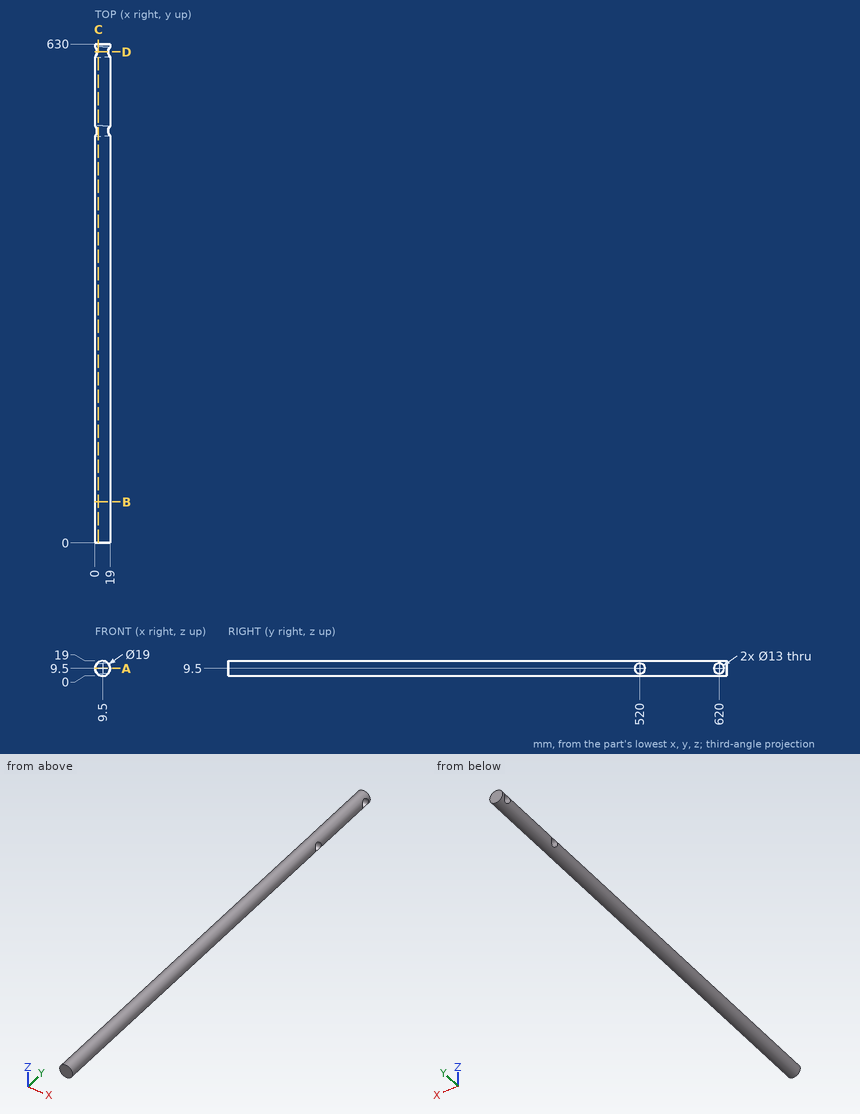
Geometry check sheet. Reference: drawing and pictorial views, mm from the part's lowest x, y, z. Round coordinates to 2 decimals unless told otherwise and drop trailing zeros. Order: outer loops, then holes, each group sorted by start corner. A loop starts at its lowest first (then second) coordinate and runs counter-clockwise, first axis right, second up. Notation, with made-up numbers: M -30.75,-0.5 L 12.25,-0.5 A24 ccw 12.25,29.5 Z; hole C -35.5,54.5 d4. An arc over 180 degrees is marked long. One line per item, written item: value. Start each with the question number.
1. Section check D-D on y = 620. Enter the section's corners in (x, z).
2. Scan lines: line 1 along Y through (x, z) = (13.25, 9.25); line 2 along Y through (x, z) = (13.5, 8.25); line 3 along X through (y, z) = (97.5, 8). Record each from-to range of solid material in increasing order.
3. Gauge pin test, flat ends, axial feed: P1, Ø6, axis at y = 226, z = 6, coming from the -X side; P2, Ø8, axis at y = 464, z = 4.5, coming from the -X side; P3, Ø1, axis at x = 3.5, y = 174.5, coming from the -Z side; P4, Ø1, axis at x = 2, z = 2.5, coming from the +Y side. Record the tip position at first contact, or that the pin passes through.
4. Section check C-C on x = 4.25. Enter the section's corners in (y, z), and give its area (3 significant figures).
5. Section check A-A on z = 9.5. Enter the section's corners in (x, y), and give its area (3 significant figures).
6. Section check B-B on y = 52. Enter the section's corners in (x, z), and give its area (3 significant figures).
Results found:
1. outline: M 2.57,3 A9.5 ccw 16.43,3 Z; M 2.57,16 L 16.43,16 A9.5 ccw Z
2. line 1: 0 to 513.5, 526.5 to 613.5, 626.5 to 630
2. line 2: 0 to 513.62, 526.38 to 613.62, 626.38 to 630
2. line 3: 0.12 to 18.88
3. P1: x = 0.01
3. P2: x = 0.05
3. P3: z = 1.75
3. P4: through
4. outline: M 0,1.58 L 630,1.58 L 630,17.42 L 0,17.42 Z; hole C 520,9.5 d13; hole C 620,9.5 d13
4. area: 9,710 mm^2
5. outline: M 0,0 L 19,0 L 19,513.5 L 0,513.5 Z; M 0,526.5 L 19,526.5 L 19,613.5 L 0,613.5 Z; M 0,626.5 L 19,626.5 L 19,630 L 0,630 Z
5. area: 11,500 mm^2
6. outline: C 9.5,9.5 d19
6. area: 284 mm^2
